CAD build for the part. Positions are in the model's coordinates, mm. A direction names the side the tool comes from. Round coordinates to 2 decimals unless told otherwise and drop trailing zeros. Loops run counter-clockwise (first coordinate to the right, second up) from the corner with the lowest first, then second, coordinate; pieces in that order, holes last.
from build123d import *

# Parameters (mm, degrees)
SKETCH1_R           = 2.5
BOSS_EXTRUDE1_DEPTH = 20
BOSS_EXTRUDE2_DEPTH = 3
FILLET1_R           = 0.5


with BuildPart() as part:
    # Sketch1 → Boss-Extrude1 (new body)
    with BuildSketch(Plane.XY):
        Circle(SKETCH1_R)
    extrude(amount=BOSS_EXTRUDE1_DEPTH)

    # Sketch3 → Boss-Extrude2 (add)
    with BuildSketch(Plane.XY.offset(20)):
        Polygon((2.782434511, 2.873683732), (-1.097465859, 3.846500837), (-3.87990037, 0.972817104), (-2.782434511, -2.873683732), (1.097465859, -3.846500837), (3.87990037, -0.972817104), align=None)
    extrude(amount=BOSS_EXTRUDE2_DEPTH)

    # Fillet1
    fillet1_edges = [part.edges().sort_by_distance(p)[0] for p in [
        (-2.5, 0, 0),
    ]]
    fillet(fillet1_edges, radius=FILLET1_R)


solid = part.part
Item 1: Wall check: L1, parallel to Z at x = -0.5, y = 3.5; L2, parallel to Y at x = -1.5, z = 11; L3, parallel to Y at x = 0, z = 5. Give the ranges that are in metal, low to high.
Verdict:
L1: z = 20 to 23
L2: y = -2 to 2
L3: y = -2.5 to 2.5
Item 2: 3-axis set-ups, long thin cutter, end or side, ignore diameter. For faces 1 (the flat face through (0, 0, 0)), 2 (the cylindrical face through (-0.54, -2.44, 10.11)): which of +Z, -Z, +X, -X, +Y, -Y reach the whole face in a straight line?
Verdict:
face 1: -Z, +X, -X, +Y, -Y
face 2: -Z
Item 3: Cut at C-C (y = 0). List the corners of the cut face in (x, z).
Verdict:
outline: (-3.6, 20) - (-2.5, 20) - (-2.5, 0.5) arc R0.5 ccw to (-2, 0) - (2, 0) arc R0.5 ccw to (2.5, 0.5) - (2.5, 20) - (3.6, 20) - (3.6, 23) - (-3.6, 23) - close
Item 4: Cut at B-B (x = 0). List the corners of the cut face in (y, z), plus the area to 3 significant figures.
Verdict:
outline: (-3.57, 20) - (-2.5, 20) - (-2.5, 0.5) arc R0.5 ccw to (-2, 0) - (2, 0) arc R0.5 ccw to (2.5, 0.5) - (2.5, 20) - (3.57, 20) - (3.57, 23) - (-3.57, 23) - close
area: 121 mm2
Item 5: Flat gauge pins, fed straight in: P1, Ø2, axis at x = -2, y = 3, coming from the -Z side; P2, Ø1, axis at y = -0.5, z = 9.5, coming from the -X side; P3, Ø1.5, axis at y = -1.5, z = 8.5, coming from the +X side. Where does each tip first touch, or does it go through?
Verdict:
P1: stops at z = 20
P2: stops at x = -2.5
P3: stops at x = 2.38
Item 6: Cut at D-D (z = 17). List the corners of the cut face in (x, y), plus the area to 3 significant figures.
Verdict:
outline: circle Ø5 at (0, 0)
area: 19.6 mm2
Item 7: Cut at A-A (z = 21). List the corners of the cut face in (x, y), plus the area to 3 significant figures.
Verdict:
outline: (-3.88, 0.97) - (-2.78, -2.87) - (1.1, -3.85) - (3.88, -0.97) - (2.78, 2.87) - (-1.1, 3.85) - close
area: 41.6 mm2
